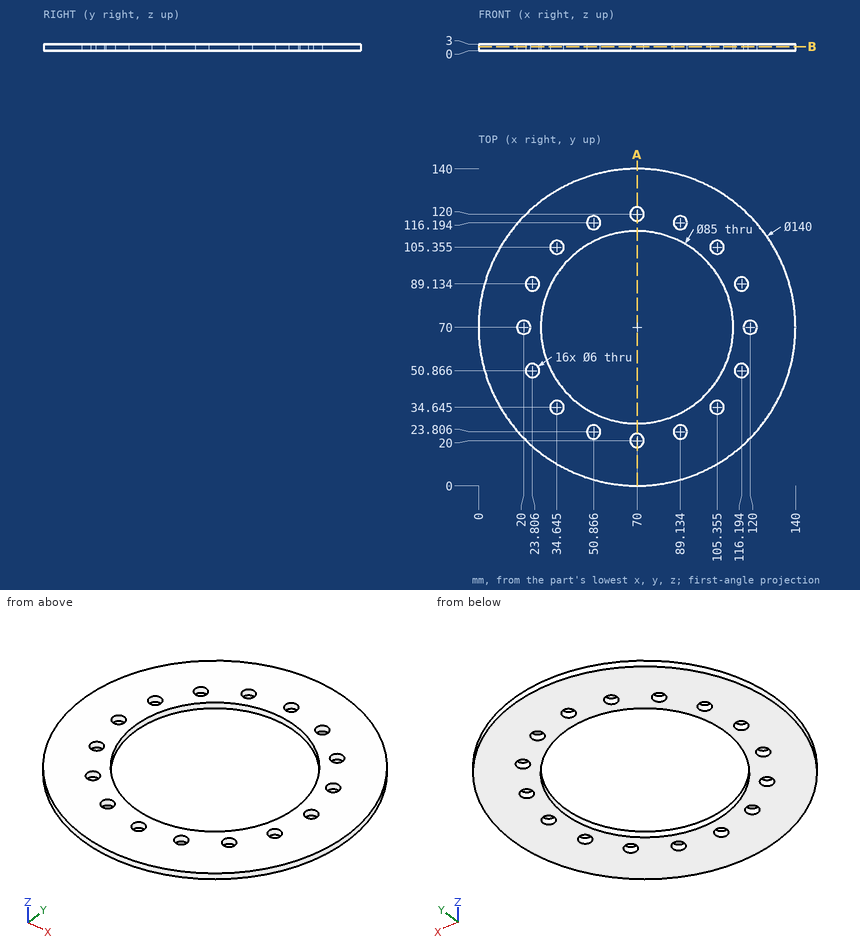
Input: dimensioned drawing with shaded views. Units: mm. Origin: part minimum x, y, z. Give positions to 0.01 mm unless a question says otherwise; leave off trailing zeros. Order: outer loops, then holes, each group sorted by start corner. A loop starts at its lowest first (then second) coordinate and runs counter-clockwise, first axis right, second up. Notation, with made-up numbers: (37.25, -23) -> (88.25, -23) arc R16 cw to (88.25, -2) -> close; hole circle Ø8 at (67.5, -40). An arc over 180 degrees is marked (long way). Use one line per item in the form item = value.
1) Line query: probe 1 along Y at (x, z) = (107, 1.1) (1 decimal); probe 2 along X at (y, z) = (90.5, 0.2) (1 decimal); probe 3 along Y at (x, z) = (36, 0.45). Output: solid intervals per line, ascending.
Response values:
probe_1 = 10.6 to 32.1, 37.2 to 49.1, 90.9 to 102.8, 107.9 to 129.4
probe_2 = 3.1 to 21.1, 26.5 to 32.8, 107.2 to 113.5, 118.9 to 136.9
probe_3 = 8.81 to 31.97, 37.32 to 44.5, 95.5 to 102.68, 108.03 to 131.19
2) Section B-B, the plane z = 1.85. Count the separate pieces of the cut face and the enclosed holes in it, and give its area (3 significant figures).
Response values:
separate_pieces = 1
enclosed_holes = 17
area = 9,270 mm^2
3) Section A-A, the plane x = 70. Return loops of the section in (y, z).
Response values:
outline = (0, 0) -> (17, 0) -> (17, 3) -> (0, 3) -> close; (23, 0) -> (27.5, 0) -> (27.5, 3) -> (23, 3) -> close; (112.5, 0) -> (117, 0) -> (117, 3) -> (112.5, 3) -> close; (123, 0) -> (140, 0) -> (140, 3) -> (123, 3) -> close
4) First-contact query: pin 1 Ø1.5 at (x, z) = (106, 0.5) entering from +Y; pin 2 Ø1 at (x, z) = (87.5, 1) entering from +Y. Flat tips, straight axial feed; report the tip coordinate or a pass-through.
Response values:
pin_1 = 130.48
pin_2 = 137.9
